The model under review builds one solid part; all positions refer to its coordinate system, in mm. Face numbers are marked on the shaded views. A direction names the side the tool comes from. Give positions to 0.01 mm unless a question says otherwise; leave off trailing zeros. Order: outer loops, then holes, each group sorted by start corner. A loop starts at its lowest first (then second) coordinate and runs counter-clockwise, first axis right, second up. Notation, with made-up numbers: (-10.5, 66) - (8.5, 66) arc R19 cw to (8.5, 94) - close; hole circle Ø4 at (-36.75, 22). An arc over 180 degrees is marked (long way). Use CSV: the item, a comma, the result in double quotes. Start each with the question number.
1. For pin 1 (5 mm diameter, centred on x = 2.5, z = 8, fed in from +Y); pin 2 (2.5 mm diameter, centred on y = 35, z = 0, fed in from -X), all flat-tipped, find the tip position at first contact; note any pin that passes through.
2. To check wall thickness, follow line 1 (Y direction, x = 21.35, z = 0); line 2 (X direction, y = 26.5, z = 8.75); line 3 (Y direction, x = 9, z = 7). State the ranges of each line that lie inside material, in increasing order. Write a range as [from, to].
3. Take a section at B-B, the plane y = 10. State the section outline as (x, z) points, then the cut area to 3 significant figures.
4. Machinability: for the marked faces 4 and 5, which of the approach directions +Z, -Z, +X, -X, +Y, -Y give a long, thin tool a straight path to every point of the face, cutting with its end or side? Answer none if there is none.
5. Draft analysis for pull direction Y (two halves, no side actions). For the marked faces 1, 2 and 3, state which applies: released by +Y, released by -Y, zero draft, split by the parting line, or undercut.
6. Take a section at D-D, the plane z = 11.5. State the section outline as (x, y) points, then the cut area to 3 significant figures.
7. Take a section at A-A, the plane y = 35. State the section outline as (x, z) points.
8. Take a section at C-C, the plane z = 0. State the section outline as (x, y) points, then the cut area to 3 significant figures.
```python
from build123d import *

# Parameters (mm, degrees)
CROQUIS1_W              = 5
CROQUIS1_H              = 28
CROQUIS1_W_2            = 40
SALIENTE_EXTRUIR1_DEPTH = 3
CROQUIS2_W              = 5
CROQUIS2_H              = 28
SALIENTE_EXTRUIR2_DEPTH = 47
CROQUIS3_R              = 1.5
CORTAR_EXTRUIR1_DEPTH   = 51


with BuildPart() as part:
    # Croquis1 → Saliente-Extruir1 (new body)
    with BuildSketch(Plane(origin=(0, 0, 0), x_dir=(1, 0, 0), z_dir=(0, 1, 0))):
        with Locations((-22.5, 0)):
            Rectangle(CROQUIS1_W, CROQUIS1_H)
        Rectangle(CROQUIS1_W_2, CROQUIS1_H)
        with Locations((22.5, 0)):
            Rectangle(CROQUIS1_W, CROQUIS1_H)
    extrude(amount=SALIENTE_EXTRUIR1_DEPTH)

    # Croquis2 → Saliente-Extruir2 (add)
    with BuildSketch(Plane(origin=(0, 3, 0), x_dir=(1, 0, 0), z_dir=(0, 1, 0))):
        with Locations((-22.5, 0)):
            Rectangle(CROQUIS2_W, CROQUIS2_H)
        with Locations((22.5, 0)):
            Rectangle(CROQUIS2_W, CROQUIS2_H)
    extrude(amount=SALIENTE_EXTRUIR2_DEPTH)

    # Croquis3 → Cortar-Extruir1 (cut, through all)
    with BuildSketch(Plane(origin=(25, 0, 0), x_dir=(0, 0, -1), z_dir=(1, 0, 0))):
        with Locations((0, 17.5)):
            Circle(CROQUIS3_R)
        with Locations((0, 35)):
            Circle(CROQUIS3_R)
    extrude(amount=-CORTAR_EXTRUIR1_DEPTH, mode=Mode.SUBTRACT)


solid = part.part
```
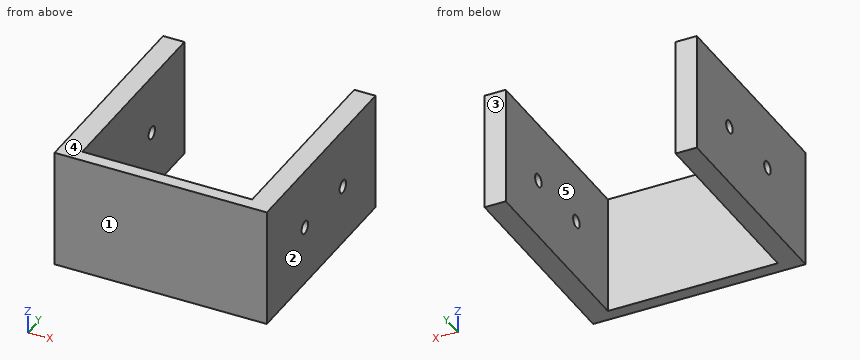
Determined:
1,pin 1,"stops at y = 3"
1,pin 2,"passes through"
2,line 1,"y = [0, 16], [19, 33.5], [36.5, 50]"
2,line 2,"x = [-25, -20], [20, 25]"
2,line 3,"y = [0, 3]"
3,outline,"(-25, -14) - (-20, -14) - (-20, 14) - (-25, 14) - close; (20, -14) - (25, -14) - (25, 14) - (20, 14) - close"
3,area,"280 mm²"
4,face 4,"+Z, +X, -X, +Y, -Y"
4,face 5,"+Z, -Z, +Y"
5,face 1,"released by -Y"
5,face 2,"zero draft"
5,face 3,"released by +Y"
6,outline,"(-25, 0) - (25, 0) - (25, 50) - (20, 50) - (20, 3) - (-20, 3) - (-20, 50) - (-25, 50) - close"
6,area,"620 mm²"
7,outline,"(-25, -14) - (-20, -14) - (-20, -1.5) - (-25, -1.5) - close; (-25, 1.5) - (-20, 1.5) - (-20, 14) - (-25, 14) - close; (20, -14) - (25, -14) - (25, -1.5) - (20, -1.5) - close; (20, 1.5) - (25, 1.5) - (25, 14) - (20, 14) - close"
8,outline,"(-25, 0) - (25, 0) - (25, 16) - (20, 16) - (20, 3) - (-20, 3) - (-20, 16) - (-25, 16) - close; (-25, 19) - (-20, 19) - (-20, 33.5) - (-25, 33.5) - close; (-25, 36.5) - (-20, 36.5) - (-20, 50) - (-25, 50) - close; (20, 19) - (25, 19) - (25, 33.5) - (20, 33.5) - close; (20, 36.5) - (25, 36.5) - (25, 50) - (20, 50) - close"
8,area,"560 mm²"
